Autodesk Inventor part; units mm, degrees
ref_plane "YZ Plane" through (0, 0, 0) normal (1, 0, 0) x (0, 1, 0)
ref_plane "XZ Plane" through (0, 0, 0) normal (0, 1, 0) x (-1, 0, 0)
ref_plane "XY Plane" through (0, 0, 0) normal (0, 0, 1) x (1, 0, 0)
sketch "Sketch1" plane through (0, 0, 0) normal (0, 1, 0) x (-1, 0, 0)
  line L0 (-9.525, -33) -> (-9.525, -22.225)
  line L1 (-9.525, 22.225) -> (-9.525, 33)
  line L2 (33, 9.525) -> (22.225, 9.525)
  line L3 (-22.225, 9.525) -> (-33, 9.525)
  line L4 (9.525, 33) -> (9.525, 22.225)
  line L5 (9.525, -22.225) -> (9.525, -33)
  line L6 (-33, -9.525) -> (-22.225, -9.525)
  line L7 (22.225, -9.525) -> (33, -9.525)
  line L8 (77.6073, 0) -> (-79.7857, 0)
  line L9 (0, -77.9019) -> (0, 71.2895)
  circle A0 centre (-35, 0) radius 2
  circle A1 centre (-22, 0) radius 2
  circle A2 centre (0, -22) radius 2
  circle A3 centre (0, -35) radius 2
  circle A4 centre (22, 0) radius 2
  circle A5 centre (35, 0) radius 2
  circle A6 centre (0, 22) radius 2
  circle A7 centre (0, 35) radius 2
  circle A8 centre (0, 0) radius 9.185
  line L10 (-57.3009, 49.9764) -> (55.1226, 49.9764) construction
  line L11 (55.1226, 49.9764) -> (55.1226, -56.5889) construction
  line L12 (55.1226, -56.5889) -> (-57.3009, -56.5889) construction
  line L13 (-57.3009, -56.5889) -> (-57.3009, 49.9764) construction
  arc A9 (9.525, 33) -> (0, 42.525) centre (0, 33) ccw
  arc A10 (0, 42.525) -> (-9.525, 33) centre (0, 33) ccw
  arc A11 (42.525, 0) -> (33, 9.525) centre (33, 0) ccw
  arc A12 (33, -9.525) -> (42.525, 0) centre (33, 0) ccw
  arc A13 (0, -42.525) -> (9.525, -33) centre (0, -33) ccw
  arc A14 (-9.525, -33) -> (0, -42.525) centre (0, -33) ccw
  arc A15 (-42.525, 0) -> (-33, -9.525) centre (-33, 0) ccw
  arc A16 (-33, 9.525) -> (-42.525, 0) centre (-33, 0) ccw
  arc A17 (9.525, 22.225) -> (22.225, 9.525) centre (22.225, 22.225) ccw
  arc A18 (22.225, -9.525) -> (9.525, -22.225) centre (22.225, -22.225) ccw
  arc A19 (-9.525, -22.225) -> (-22.225, -9.525) centre (-22.225, -22.225) ccw
  arc A20 (-22.225, 9.525) -> (-9.525, 22.225) centre (-22.225, 22.225) ccw
  point P0 (0, 42.525)
  point P1 (42.525, 0)
  point P2 (0, -42.525)
  point P3 (-42.525, 0)
  point P4 (42.525, 0)
  point P5 (0, 42.525)
  point P6 (-42.525, 0)
  dimension "d2" = 360
  dimension "d4" = 4
  dimension "d5" = 22
  dimension "d6" = 35
  dimension "d7" = 18.37
  dimension "d39" = 9.525
  dimension "d41" = 9.525
  dimension "d46" = 12.7
extrude "Extrusion1" add sketch "Sketch1" along normal blind 4 contours L0 A19 L6 A15 L8 A0 A1 A8 L9 A2 A3 A14 | L9 A3 A2 A8 L8 A4 A5 A12 L7 A18 L5 A13 | A16 L3 A20 L1 A10 L9 A7 A6 A8 L8 A1 A0 | L8 A5 A4 A8 L9 A6 A7 A9 L4 A17 L2 A11
properties part number "DriveMotorPlate"
Check sheet for the modelled part. Datum: model origin and axes. Units: mm. A direction names the side the tool comes from. Round coordinates to 2 decimals unless told otherwise and drop trailing zeros. Write each loop counter-clockwise with the first axis right and the second up, starting at its lowest first coordinate (ties: lowest second). Pieces come first, ordered by that corner, then holes. Notation, with made-up numbers: (-20.5, 33.5) -> (3.5, 33.5) arc R21 cw to (3.5, 61.5) -> close; hole circle Ø5 at (59.25, 87). An arc over 180 degrees is marked (long way). One line per question, with ' | ' between items. Start each with the question number.
1. Scan lines: line 1 along Z through (x, y) = (0, 1.4) (3 decimals); line 2 along Z through (x, y) = (-22, 2.75). Record each from-to range of solid material in increasing order. Write a range as from..to.
2. Sectioned sample at B-B, the plane x = 0. Record the cut outline in (y, z) (3 decimals), then the cut area to 3 significant figures.
3. Depth check by flat-ended pin: pin 1 (2 mm diameter, centred on x = -25, y = 1.5, fed in from +Z) (3 decimals); pin 2 (6.5 mm diameter, centred on x = -35, z = 0, fed in from +Y); pin 3 (2 mm diameter, centred on y = 3.5, z = -1.5, fed in from +X); pin 4 (3 mm diameter, centred on x = 22, z = 0, fed in from -Y) (3 decimals). Enter the tip coordinate at first touch or a pass-through.
4. Sectioned sample at C-C, the plane y = 1. Count the separate pieces of the cut face and the enclosed holes in it, then the cut area to 3 significant figures.
5. Sectioned sample at A-A, the plane z = 0. Record the cut outline in (x, y) (3 decimals), then the cut area to 3 significant figures.
6. Sectioned sample at D-D, the plane z = 35. Record the cut outline in (x, y).
7. Release check for a two-part mould opening along Z. For faces 1 (the face through (0, 2, 37)), 2 (the face through (-9.525, 2, 28)), 3 (the face through (-36.847, 1.972, 0.766)), 4 (the face through (-13.15, 1.97, -13.34)) record: +Z half, -Z half, draft (parallel to the pull), parting line (faces both ways), or undercut.
8. Set-up check for faces 5 (the face through (9.525, 2, -28)), 6 (the face through (-42.523, 1.972, 0.209)), 7 (the face through (-9.525, 2, -28)), 8 (the face through (0, 2, -33)), 9 (the face through (28, 2, 9.525)): record each of +Z, -Z, +X, -X, +Y, -Y from which the full face is reachable in a straight line by a thin tool's end or side.
Taken from the geometry:
1) line 1: z = -42.525..-37, -33..-24, -20..-9.185, 9.185..20, 24..33, 37..42.525 | line 2: z = -9.53..-2, 2..9.53
2) outline: (0, -42.525) -> (4, -42.525) -> (4, -37) -> (0, -37) -> close; (0, -33) -> (4, -33) -> (4, -24) -> (0, -24) -> close; (0, -20) -> (4, -20) -> (4, -9.185) -> (0, -9.185) -> close; (0, 9.185) -> (4, 9.185) -> (4, 20) -> (0, 20) -> close; (0, 24) -> (4, 24) -> (4, 33) -> (0, 33) -> close; (0, 37) -> (4, 37) -> (4, 42.525) -> (0, 42.525) -> close | area: 203 mm^2
3) pin 1: stops at z = 9.525 | pin 2: stops at y = 4 | pin 3: stops at x = 42.51 | pin 4: passes through
4) separate pieces: 1 | enclosed holes: 9 | area: 2,490 mm^2
5) outline: (-42.525, 0) -> (-37, 0) -> (-37, 4) -> (-42.525, 4) -> close; (-33, 0) -> (-24, 0) -> (-24, 4) -> (-33, 4) -> close; (-20, 0) -> (-9.185, 0) -> (-9.185, 4) -> (-20, 4) -> close; (9.185, 0) -> (20, 0) -> (20, 4) -> (9.185, 4) -> close; (24, 0) -> (33, 0) -> (33, 4) -> (24, 4) -> close; (37, 0) -> (42.525, 0) -> (42.525, 4) -> (37, 4) -> close | area: 203 mm^2
6) outline: (-9.31, 0) -> (-2, 0) -> (-2, 4) -> (-9.31, 4) -> close; (2, 0) -> (9.31, 0) -> (9.31, 4) -> (2, 4) -> close
7) face 1: undercut | face 2: draft | face 3: undercut | face 4: -Z half
8) face 5: -Z, +X, +Y, -Y | face 6: -X, +Y, -Y | face 7: -Z, -X, +Y, -Y | face 8: +Y, -Y | face 9: +Z, +X, +Y, -Y
